The model under review builds one solid part; all positions refer to its coordinate system, in mm. Face numbers are marked on the shaded views. Round coordinates to 2 decimals unless told otherwise and drop trailing zeros. Loops run counter-clockwise (first coordinate to the right, second up) from the corner with the lowest first, then second, coordinate; pieces in that order, holes last. Notation, with made-up numbers: (-14, 49) -> (34, 49) arc R18 cw to (34, 68) -> close; hole circle Ø4 at (38, 20.5). An arc over 180 degrees is marked (long way). Write each question's results on one line, items separated by ' | '. Start each with the question number.
Item 1: Mouldability with a two-part tool opening along Z and no side actions: class the marked faces 1, 2, 3 and 4 as pulls with the +Z half, pulls with the -Z half, needs draft (parallel to the pull), parting line crosses it, or undercut.
Item 2: We need section A-A (z = 540). Give the boundary of the cut face in (x, y), and give its area (3 significant figures).
Item 3: Clearance check with flat-ended pins moving along their axes: pin 1 Ø3 at (x, z) = (-24.5, 146) entering from -Y; pin 2 Ø6 at (x, z) = (11, 172) entering from -Y; pin 3 Ø4 at (y, z) = (-40.5, 243) entering from +X. State where each tip first meets the part, or that it passes through.
Item 4: We need section B-B (z = 443.5). Give the boundary of the cut face in (x, y), and give its area (3 significant figures).
Item 5: For L1, parallel to Y at x = 0, z = 6; L2, parallel to Z at x = -52.5, y = 45.5; L3, parallel to Z at x = 2, y = -23, list the stretches that pass through material, from the lowest coordinate up. Write a range as from..to.
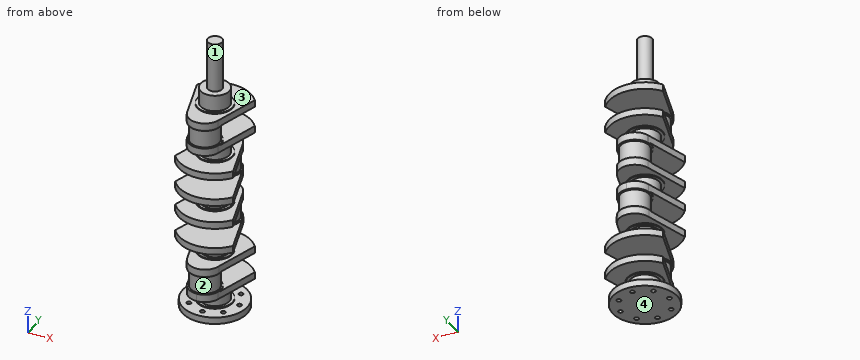
from build123d import *

# Parameters (mm, degrees)
SKETCH1_R            = 72
SKETCH1_R_2          = 5
BOSS_EXTRUDE1_DEPTH  = 15
SKETCH2_R            = 39
BOSS_EXTRUDE2_DEPTH  = 2
SKETCH3_R            = 32
BOSS_EXTRUDE3_DEPTH  = 36
SKETCH4_R            = 80
BOSS_EXTRUDE4_DEPTH  = 15.5
CUT_EXTRUDE2_DEPTH   = 15.5
SKETCH7_R            = 39
SKETCH7_R_2          = 32
BOSS_EXTRUDE6_DEPTH  = 2
SKETCH9_R            = 36
BOSS_EXTRUDE7_DEPTH  = 2
SKETCH10_R           = 32
BOSS_EXTRUDE8_DEPTH  = 41
SKETCH11_R           = 36
BOSS_EXTRUDE9_DEPTH  = 2
BOSS_EXTRUDE10_DEPTH = 15.5
SKETCH14_R           = 39
BOSS_EXTRUDE11_DEPTH = 2
SKETCH15_R           = 32
BOSS_EXTRUDE12_DEPTH = 34
SKETCH16_R           = 39
BOSS_EXTRUDE13_DEPTH = 2
BOSS_EXTRUDE14_DEPTH = 15.5
SKETCH18_R           = 36
BOSS_EXTRUDE15_DEPTH = 2
SKETCH19_R           = 32
BOSS_EXTRUDE16_DEPTH = 41
SKETCH20_R           = 36
BOSS_EXTRUDE17_DEPTH = 2
BOSS_EXTRUDE18_DEPTH = 15.5
SKETCH22_R           = 39
BOSS_EXTRUDE19_DEPTH = 2
SKETCH23_R           = 32
BOSS_EXTRUDE20_DEPTH = 34
SKETCH24_R           = 39
BOSS_EXTRUDE21_DEPTH = 2
BOSS_EXTRUDE22_DEPTH = 15.5
SKETCH29_R           = 36
BOSS_EXTRUDE26_DEPTH = 2
SKETCH30_R           = 32
BOSS_EXTRUDE27_DEPTH = 41
SKETCH31_R           = 36
BOSS_EXTRUDE28_DEPTH = 2
BOSS_EXTRUDE29_DEPTH = 15.5
SKETCH33_R           = 39
BOSS_EXTRUDE30_DEPTH = 2
SKETCH34_R           = 32
BOSS_EXTRUDE31_DEPTH = 34
SKETCH35_R           = 39
BOSS_EXTRUDE32_DEPTH = 2
BOSS_EXTRUDE33_DEPTH = 15.5
SKETCH37_R           = 36
BOSS_EXTRUDE34_DEPTH = 2
SKETCH38_R           = 32
BOSS_EXTRUDE35_DEPTH = 41
SKETCH39_R           = 36
BOSS_EXTRUDE36_DEPTH = 2
BOSS_EXTRUDE37_DEPTH = 15.5
SKETCH43_R           = 39
BOSS_EXTRUDE38_DEPTH = 2
SKETCH44_R           = 32
BOSS_EXTRUDE39_DEPTH = 36
SKETCH45_R           = 16
BOSS_EXTRUDE40_DEPTH = 110


with BuildPart() as part:
    # Sketch1 → Boss-Extrude1 (new body)
    with BuildSketch(Plane.XY):
        Circle(SKETCH1_R)
        with Locations((0, 54.5)):
            Circle(SKETCH1_R_2, mode=Mode.SUBTRACT)
        with Locations((38.537319575, 38.537319575)):
            Circle(SKETCH1_R_2, mode=Mode.SUBTRACT)
        with Locations((54.5, 0)):
            Circle(SKETCH1_R_2, mode=Mode.SUBTRACT)
        with Locations((38.537319575, -38.537319575)):
            Circle(SKETCH1_R_2, mode=Mode.SUBTRACT)
        with Locations((0, -54.5)):
            Circle(SKETCH1_R_2, mode=Mode.SUBTRACT)
        with Locations((-38.537319575, -38.537319575)):
            Circle(SKETCH1_R_2, mode=Mode.SUBTRACT)
        with Locations((-54.5, 0)):
            Circle(SKETCH1_R_2, mode=Mode.SUBTRACT)
        with Locations((-38.537319575, 38.537319575)):
            Circle(SKETCH1_R_2, mode=Mode.SUBTRACT)
    extrude(amount=BOSS_EXTRUDE1_DEPTH)

    # Sketch2 → Boss-Extrude2 (add)
    with BuildSketch(Plane.XY.offset(15)):
        Circle(SKETCH2_R)
    extrude(amount=BOSS_EXTRUDE2_DEPTH)

    # Sketch3 → Boss-Extrude3 (add)
    with BuildSketch(Plane.XY.offset(17)):
        Circle(SKETCH3_R)
    extrude(amount=BOSS_EXTRUDE3_DEPTH)

    # Sketch4 → Boss-Extrude4 (add)
    with BuildSketch(Plane.XY.offset(53)):
        Circle(SKETCH4_R)
    extrude(amount=BOSS_EXTRUDE4_DEPTH)

    # Sketch5 → Cut-Extrude2 (cut)
    with BuildSketch(Plane.XY.offset(68.5)):
        with BuildLine():
            ThreePointArc((-7.7e-08, -80), (-21.539685652, -72.845137234), (-34.517510455, -54.224552409))
            Line((-34.517510455, -54.224552409), (-64.569893475, 47.23059238))
            ThreePointArc((-64.569893475, 47.23059238), (-71.33879518, -36.204644761), (-7.7e-08, -80))
        make_face()
        with BuildLine():
            ThreePointArc((34.517510455, -54.224552409), (21.53968559, -72.84513728), (-7.7e-08, -80))
            ThreePointArc((-7.7e-08, -80), (56.568542468, -56.568542522), (80, 0))
            ThreePointArc((80, 0), (76.044695667, 24.843595975), (64.569893475, 47.23059238))
            Line((64.569893475, 47.23059238), (34.517510455, -54.224552409))
        make_face()
    extrude(amount=-CUT_EXTRUDE2_DEPTH, mode=Mode.SUBTRACT)

    # Sketch7 → Boss-Extrude6 (add)
    with BuildSketch(Plane(origin=(0, 0, 53), x_dir=(-1, 0, 0), z_dir=(0, 0, -1))):
        Circle(SKETCH7_R)
        Circle(SKETCH7_R_2, mode=Mode.SUBTRACT)
    extrude(amount=BOSS_EXTRUDE6_DEPTH)

    # Sketch9 → Boss-Extrude7 (add)
    with BuildSketch(Plane.XY.offset(68.5)):
        with Locations((0, -44)):
            Circle(SKETCH9_R)
    extrude(amount=BOSS_EXTRUDE7_DEPTH)

    # Sketch10 → Boss-Extrude8 (add)
    with BuildSketch(Plane.XY.offset(70.5)):
        with Locations((0, -44)):
            Circle(SKETCH10_R)
    extrude(amount=BOSS_EXTRUDE8_DEPTH)

    # Sketch11 → Boss-Extrude9 (add)
    with BuildSketch(Plane.XY.offset(111.5)):
        with Locations((0, -44)):
            Circle(SKETCH11_R)
    extrude(amount=BOSS_EXTRUDE9_DEPTH)

    # Sketch13 → Boss-Extrude10 (add)
    with BuildSketch(Plane.XY.offset(113.5)):
        with BuildLine():
            Line((-64.569893475, 47.23059238), (-35.103878052, -51.982339614))
            ThreePointArc((-35.103878052, -51.982339614), (0.703146821, -79.993132464), (35.38885459, -50.605222996))
            Line((35.38885459, -50.605222996), (64.569893475, 47.23059238))
            ThreePointArc((64.569893475, 47.23059238), (0, 80), (-64.569893475, 47.23059238))
        make_face()
    extrude(amount=BOSS_EXTRUDE10_DEPTH)

    # Sketch14 → Boss-Extrude11 (add)
    with BuildSketch(Plane.XY.offset(129)):
        Circle(SKETCH14_R)
    extrude(amount=BOSS_EXTRUDE11_DEPTH)

    # Sketch15 → Boss-Extrude12 (add)
    with BuildSketch(Plane.XY.offset(131)):
        Circle(SKETCH15_R)
    extrude(amount=BOSS_EXTRUDE12_DEPTH)

    # Sketch16 → Boss-Extrude13 (add)
    with BuildSketch(Plane.XY.offset(165)):
        Circle(SKETCH16_R)
    extrude(amount=BOSS_EXTRUDE13_DEPTH)

    # Sketch17 → Boss-Extrude14 (add)
    with BuildSketch(Plane.XY.offset(167)):
        with BuildLine():
            Line((-64.569893475, -47.23059238), (-35.103878052, 51.982339614))
            ThreePointArc((-35.103878052, 51.982339614), (0.703146821, 79.993132464), (35.38885459, 50.605222996))
            Line((35.38885459, 50.605222996), (64.569893475, -47.23059238))
            ThreePointArc((64.569893475, -47.23059238), (0, -80), (-64.569893475, -47.23059238))
        make_face()
    extrude(amount=BOSS_EXTRUDE14_DEPTH)

    # Sketch18 → Boss-Extrude15 (add)
    with BuildSketch(Plane.XY.offset(182.5)):
        with Locations((0, 44)):
            Circle(SKETCH18_R)
    extrude(amount=BOSS_EXTRUDE15_DEPTH)

    # Sketch19 → Boss-Extrude16 (add)
    with BuildSketch(Plane.XY.offset(184.5)):
        with Locations((0, 44)):
            Circle(SKETCH19_R)
    extrude(amount=BOSS_EXTRUDE16_DEPTH)

    # Sketch20 → Boss-Extrude17 (add)
    with BuildSketch(Plane.XY.offset(225.5)):
        with Locations((0, 44)):
            Circle(SKETCH20_R)
    extrude(amount=BOSS_EXTRUDE17_DEPTH)

    # Sketch21 → Boss-Extrude18 (add)
    with BuildSketch(Plane.XY.offset(227.5)):
        with BuildLine():
            Line((-34.94290999, 52.659852274), (-64.569893475, -47.23059238))
            ThreePointArc((-64.569893475, -47.23059238), (0, -80), (64.569893475, -47.23059238))
            Line((64.569893475, -47.23059238), (34.517510455, 54.224552409))
            ThreePointArc((34.517510455, 54.224552409), (35.627449926, 49.165734392), (36, 44))
            ThreePointArc((36, 44), (-4.362066044, 8.265249688), (-34.94290999, 52.659852274))
        make_face()
        with BuildLine():
            ThreePointArc((0, 80), (-22.183837789, 72.352730749), (-34.94290999, 52.659852274))
            ThreePointArc((-34.94290999, 52.659852274), (-4.362066044, 8.265249688), (36, 44))
            ThreePointArc((36, 44), (35.627449926, 49.165734392), (34.517510455, 54.224552409))
            ThreePointArc((34.517510455, 54.224552409), (21.539685621, 72.845137257), (0, 80))
        make_face()
    extrude(amount=BOSS_EXTRUDE18_DEPTH)

    # Sketch22 → Boss-Extrude19 (add)
    with BuildSketch(Plane.XY.offset(243)):
        Circle(SKETCH22_R)
    extrude(amount=BOSS_EXTRUDE19_DEPTH)

    # Sketch23 → Boss-Extrude20 (add)
    with BuildSketch(Plane.XY.offset(245)):
        Circle(SKETCH23_R)
    extrude(amount=BOSS_EXTRUDE20_DEPTH)

    # Sketch24 → Boss-Extrude21 (add)
    with BuildSketch(Plane.XY.offset(279)):
        Circle(SKETCH24_R)
    extrude(amount=BOSS_EXTRUDE21_DEPTH)

    # Sketch25 → Boss-Extrude22 (add)
    with BuildSketch(Plane.XY.offset(281)):
        with BuildLine():
            Line((64.569893475, -47.23059238), (34.517510455, 54.224552409))
            ThreePointArc((34.517510455, 54.224552409), (0, 80), (-34.517510455, 54.224552409))
            Line((-34.517510455, 54.224552409), (-64.569893475, -47.23059238))
            ThreePointArc((-64.569893475, -47.23059238), (0, -80), (64.569893475, -47.23059238))
        make_face()
    extrude(amount=BOSS_EXTRUDE22_DEPTH)

    # Sketch29 → Boss-Extrude26 (add)
    with BuildSketch(Plane.XY.offset(296.5)):
        with Locations((0, 44)):
            Circle(SKETCH29_R)
    extrude(amount=BOSS_EXTRUDE26_DEPTH)

    # Sketch30 → Boss-Extrude27 (add)
    with BuildSketch(Plane.XY.offset(298.5)):
        with Locations((0, 44)):
            Circle(SKETCH30_R)
    extrude(amount=BOSS_EXTRUDE27_DEPTH)

    # Sketch31 → Boss-Extrude28 (add)
    with BuildSketch(Plane.XY.offset(339.5)):
        with Locations((0, 44)):
            Circle(SKETCH31_R)
    extrude(amount=BOSS_EXTRUDE28_DEPTH)

    # Sketch32 → Boss-Extrude29 (add)
    with BuildSketch(Plane.XY.offset(341.5)):
        with BuildLine():
            Line((-35.001162126, 52.421321146), (-64.569893475, -47.23059238))
            ThreePointArc((-64.569893475, -47.23059238), (0, -80), (64.569893475, -47.23059238))
            Line((64.569893475, -47.23059238), (34.517510455, 54.224552409))
            ThreePointArc((34.517510455, 54.224552409), (0.950243427, 79.987456668), (-33.929832299, 56.031894288))
            Line((-33.929832299, 56.031894288), (-35.001162126, 52.421321146))
        make_face()
    extrude(amount=BOSS_EXTRUDE29_DEPTH)

    # Sketch33 → Boss-Extrude30 (add)
    with BuildSketch(Plane.XY.offset(357)):
        Circle(SKETCH33_R)
    extrude(amount=BOSS_EXTRUDE30_DEPTH)

    # Sketch34 → Boss-Extrude31 (add)
    with BuildSketch(Plane.XY.offset(359)):
        Circle(SKETCH34_R)
    extrude(amount=BOSS_EXTRUDE31_DEPTH)

    # Sketch35 → Boss-Extrude32 (add)
    with BuildSketch(Plane.XY.offset(393)):
        Circle(SKETCH35_R)
    extrude(amount=BOSS_EXTRUDE32_DEPTH)

    # Sketch36 → Boss-Extrude33 (add)
    with BuildSketch(Plane.XY.offset(395)):
        with BuildLine():
            Line((-64.569893475, 47.23059238), (-35.103878052, -51.982339614))
            ThreePointArc((-35.103878052, -51.982339614), (-1.158808135, -79.981344662), (34.517510455, -54.224552409))
            Line((34.517510455, -54.224552409), (64.569893475, 47.23059238))
            ThreePointArc((64.569893475, 47.23059238), (0, 80), (-64.569893475, 47.23059238))
        make_face()
    extrude(amount=BOSS_EXTRUDE33_DEPTH)

    # Sketch37 → Boss-Extrude34 (add)
    with BuildSketch(Plane.XY.offset(410.5)):
        with Locations((0, -44)):
            Circle(SKETCH37_R)
    extrude(amount=BOSS_EXTRUDE34_DEPTH)

    # Sketch38 → Boss-Extrude35 (add)
    with BuildSketch(Plane.XY.offset(412.5)):
        with Locations((0, -44)):
            Circle(SKETCH38_R)
    extrude(amount=BOSS_EXTRUDE35_DEPTH)

    # Sketch39 → Boss-Extrude36 (add)
    with BuildSketch(Plane.XY.offset(453.5)):
        with Locations((0, -44)):
            Circle(SKETCH39_R)
    extrude(amount=BOSS_EXTRUDE36_DEPTH)

    # Sketch42 → Boss-Extrude37 (add)
    with BuildSketch(Plane.XY.offset(455.5)):
        with BuildLine():
            Line((-64.569893475, 47.23059238), (-35.103878052, -51.982339614))
            ThreePointArc((-35.103878052, -51.982339614), (-1.158808135, -79.981344662), (34.517510455, -54.224552409))
            Line((34.517510455, -54.224552409), (64.569893475, 47.23059238))
            ThreePointArc((64.569893475, 47.23059238), (0, 80), (-64.569893475, 47.23059238))
        make_face()
    extrude(amount=BOSS_EXTRUDE37_DEPTH)

    # Sketch43 → Boss-Extrude38 (add)
    with BuildSketch(Plane.XY.offset(471)):
        Circle(SKETCH43_R)
    extrude(amount=BOSS_EXTRUDE38_DEPTH)

    # Sketch44 → Boss-Extrude39 (add)
    with BuildSketch(Plane.XY.offset(473)):
        Circle(SKETCH44_R)
    extrude(amount=BOSS_EXTRUDE39_DEPTH)

    # Sketch45 → Boss-Extrude40 (add)
    with BuildSketch(Plane.XY.offset(509)):
        Circle(SKETCH45_R)
    extrude(amount=BOSS_EXTRUDE40_DEPTH)


solid = part.part
Here are the results:
1) face 1: needs draft | face 2: undercut | face 3: pulls with the +Z half | face 4: pulls with the -Z half
2) outline: circle Ø32 at (0, 0) | area: 804 mm2
3) pin 1: stops at y = -22.25 | pin 2: stops at y = -79.6 | pin 3: stops at x = 63.17
4) outline: circle Ø64 at (0, -44) | area: 3,220 mm2
5) L1: y = -72..-59.5, -49.5..49.5, 59.5..72 | L2: z = 0..15, 53..68.5, 113.5..129, 395..410.5, 455.5..471 | L3: z = 0..182.5, 227.5..296.5, 341.5..509
